from build123d import *

# Parameters (mm, degrees)
F1_DEPTH         = 19
F0_W             = 44.0000004768
F0_H             = 45.5000002384
F0_R             = 12
F2_DEPTH         = 2
F3_D             = 4
F5_DEPTH         = 50
F7_DEPTH         = 3
F8_D             = 4
F9_R             = 2
F10_R            = 34.4476203659
F10_W            = 47
F10_H            = 19
F6_W             = 47
F6_H             = 19
F11_DEPTH        = 3
F13_DEPTH        = 25
F14_D            = 4
F14_DEPTH        = 6
F14_TIP          = 1.2017212381
F14_ON_F12_D     = 4
F14_ON_F12_DEPTH = 6
F14_ON_F12_TIP   = 1.2017212381


# Not quite as in the source:
# - a feature names something its author has since deleted; it is built from what else it names


with BuildPart() as f1:
    # F0 (on Top) → F1 (new body)
    with BuildSketch(Plane.XY):
        Polygon((23.5, -23.5), (23.5, 23.5), (-23.5, 23.5), (-23.5, -23.5), (-22.0000002384, -23.5), (-22.0000002384, 22.0000002384), (22.0000002384, 22.0000002384), (22.0000002384, -23.5), align=None)
    extrude(amount=F1_DEPTH)

    # F0 (on Top) → F2 (join)
    with BuildSketch(Plane.XY):
        with Locations((0, -0.7499998808)):
            Rectangle(F0_W, F0_H)
        Circle(F0_R, mode=Mode.SUBTRACT)
    extrude(amount=F2_DEPTH)

    # F3 (through all)
    with Locations(Plane(origin=(0, 0, 0), x_dir=(1, 0, 0), z_dir=(0, 0, -1))):
        with Locations((-15.5, -15.5), (15.5, -15.5), (15.5, 15.5), (-15.5, 15.5)):
            Hole(F3_D / 2)

    # F4 (on face) → F5 (cut)
    with BuildSketch(Plane.YZ.offset(23.5)):
        Polygon((-23.5, 19), (-23.5, 2.1775800269), (17.5668895245, 19), align=None)
    extrude(amount=-F5_DEPTH, mode=Mode.SUBTRACT)

    # F6 (on face) → F7 (join)
    with BuildSketch(Plane(origin=(0, 23.5, 0), x_dir=(-1, 0, 0), z_dir=(0, 1, 0))):
        with BuildLine():
            Line((-23.5, 19), (-25.1444590574, 19))
            ThreePointArc((-25.1444590574, 19), (-28.6799929633, 17.5355339059), (-30.1444590574, 14))
            Line((-30.1444590574, 14), (-30.1444590574, 5))
            ThreePointArc((-30.1444590574, 5), (-28.6799929633, 1.4644660941), (-25.1444590574, 0))
            Line((-25.1444590574, 0), (-23.5, 0))
            Line((-23.5, 0), (-23.5, 19))
        make_face()
        with BuildLine():
            Line((24.0855421871, 19), (23.5, 19))
            Line((23.5, 19), (23.5, 0))
            Line((23.5, 0), (24.0855421871, 0))
            ThreePointArc((24.0855421871, 0), (27.621076093, 1.4644660941), (29.0855421871, 5))
            Line((29.0855421871, 5), (29.0855421871, 14))
            ThreePointArc((29.0855421871, 14), (27.621076093, 17.5355339059), (24.0855421871, 19))
        make_face()
    extrude(amount=-F7_DEPTH)

    # F8 (through all)
    with Locations(Plane(origin=(0, 23.5, 0), x_dir=(-1, 0, 0), z_dir=(0, 1, 0))):
        with Locations((-26.7366040498, 8.9737372473), (28.2633959502, 9.5)):
            Hole(F8_D / 2)

    # F9
    f9_edges = [f1.edges().sort_by_distance(p)[0] for p in [
        (22, 22, 10.5),
        (-22, 22, 10.5),
    ]]
    fillet(f9_edges, radius=F9_R)

    # F10 (on face) + F6 (on face) → F11 (join)
    with BuildSketch(Plane(origin=(0, 23.5, 0), x_dir=(-1, 0, 0), z_dir=(0, 1, 0))):
        with Locations((0, 19.7549201548)):
            Circle(F10_R)
        with Locations((0, 9.5)):
            Rectangle(F10_W, F10_H, mode=Mode.SUBTRACT)
    with BuildSketch(Plane(origin=(0, 23.5, 0), x_dir=(-1, 0, 0), z_dir=(0, 1, 0))):
        with Locations((0, 9.5)):
            Rectangle(F6_W, F6_H)
    extrude(amount=-F11_DEPTH)

    # F12 (on face) → F13 (cut)
    with BuildSketch(Plane(origin=(0, 23.5, 0), x_dir=(-1, 0, 0), z_dir=(0, 1, 0))):
        with BuildLine():
            ThreePointArc((-18.1099253817, 36.3759554919), (-20.9291093364, 32.8831264718), (-21.9364919731, 28.5090170817))
            Line((-21.9364919731, 28.5090170817), (-21.9364919731, 14.7631261498))
            Line((-21.9364919731, 14.7631261498), (21.9364919731, 14.7631261498))
            Line((21.9364919731, 14.7631261498), (21.9364919731, 28.5090170817))
            ThreePointArc((21.9364919731, 28.5090170817), (20.9291093364, 32.8831264718), (18.1099253817, 36.3759554919))
            Line((18.1099253817, 36.3759554919), (6.1734334086, 45.7428952702))
            ThreePointArc((6.1734334086, 45.7428952702), (0, 47.87595686), (-6.1734334086, 45.7428952702))
            Line((-6.1734334086, 45.7428952702), (-18.1099253817, 36.3759554919))
        make_face()
        with BuildLine():
            Line((28.2202352675, 0), (-28.2202352675, 0))
            ThreePointArc((-28.2202352675, 0), (0, -14.6927002111), (28.2202352675, 0))
        make_face()
    extrude(amount=-F13_DEPTH, mode=Mode.SUBTRACT)

    # F14
    with Locations(Plane(origin=(0, 23.5, 0), x_dir=(-1, 0, 0), z_dir=(0, 1, 0))):
        with Locations((-30.1444590574, 19), (-26.7366040498, 8.9737372473), (26.7366040498, 8.9737372473), (30.1444590574, 19)):
            Hole(F14_D / 2, depth=F14_DEPTH)
            with Locations((0, 0, -(F14_DEPTH + F14_TIP / 2))):  # 118° drill point
                Cone(0, F14_D / 2, F14_TIP, mode=Mode.SUBTRACT)

    # F14 on F12
    with Locations(Plane(origin=(0, 23.5, 0), x_dir=(-1, 0, 0), z_dir=(0, 1, 0))):
        with Locations((9.4067957252, 48.2378602028), (-9.4067957252, 48.2378602028)):
            Hole(F14_ON_F12_D / 2, depth=F14_ON_F12_DEPTH)
            with Locations((0, 0, -(F14_ON_F12_DEPTH + F14_ON_F12_TIP / 2))):  # 118° drill point
                Cone(0, F14_ON_F12_D / 2, F14_ON_F12_TIP, mode=Mode.SUBTRACT)


solid = f1.part
The model under review builds one solid part; all positions refer to its coordinate system, in mm. A direction names the side the tool comes from. Give positions to 0.01 mm unless a question says otherwise; leave off trailing zeros. Write each loop counter-clockwise with the first axis right and the second up, starting at its lowest first coordinate (ties: lowest second). Pieces come first, ordered by that corner, then holes. Notation, with made-up numbers: M 78,82.25 L 123,82.25 A23 ccw 123,99.25 Z; hole C -30,-3 d7. An arc over 180 degrees is marked long. One line per question, with ' | ' between items. Start each with the question number.
Item 1: We need section D-D on z = 24.5. Write out the cut boundary in (x, y).
Item 2: Wall thickness on line 1 (Y direction, x = -15.5, z = 0.45); line 2 (Y direction, x = -23.5, z = 39); line 3 (Z direction, x = -2, y = -18): over which ranges is each line inside the solid? List them lowest first. Write a range as from..to.
Item 3: For faces 3 (the flat face through (-5.2, -11, 2)), 4 (the cylindrical face through (-15.24, 13.517, 1.014)), 5 (the flat face through (0, -23.5, 1)), 6 (the flat face through (-23, 19, 19)), 7 (the cylindrical face through (-20.957, 22.021, 32.826)), list the 3-axis set-ups (+Z, -Z, +X, -X, +Y, -Y) from which the entire face can be reached by the end or side of a thin tool; tool diameter is ignored.
Item 4: For pin 1 (5 mm diameter, centred on x = -30.14, z = 19, fed in from -Y); pin 2 (15 mm diameter, centred on y = -8, z = 11, fed in from -X); pin 3 (21 mm diameter, centred on y = 1.5, z = 12.5, fed in from +X); pin 4 (2.5 mm diameter, centred on x = 15.5, y = -15.5, fed in from +Z), all flat-tipped, find the tip position at first contact; note any pin that passes through.
Item 5: We need section C-C on x = -19.5. Write out the cut boundary in (y, z), plus the area to 3 significant figures.
Item 6: Draft analysis for pull direction X (two halves, no side actions). For faces 1 (the flat face through (0, 23.5, 9)), 2 (the cylindrical face through (-11.99, 0.53, 0.99)), state which applies: released by +X, released by -X, zero draft, split by the parting line, or undercut.
Item 7: We need section B-B on y = -2. Write out the cut boundary in (x, z).
Item 8: We need section A-A on x = 0. Write out the cut boundary in (y, z).
Results found:
1) outline: M -34.12,20.5 L -21.94,20.5 L -21.94,23.5 L -34.12,23.5 Z; M 21.94,20.5 L 34.12,20.5 L 34.12,23.5 L 21.94,23.5 Z
2) line 1: y = -23.5..-17.5, -13.5..13.5, 17.5..23.5 | line 2: y = 20.5..23.5 | line 3: z = 0..2
3) face 3: +Z, -Y | face 4: +Z, -Z | face 5: +Z, -Z, +X, -X, -Y | face 6: +Z, +X, -X, -Y | face 7: +Y, -Y
4) pin 1: stops at y = 20.5 | pin 2: stops at x = -23.5 | pin 3: stops at x = 23.5 | pin 4: passes through
5) outline: M -23.5,0 L 23.5,0 L 23.5,14.76 L 20.5,14.76 L 20.5,2 L -23.5,2 Z; M 20.5,35.05 L 23.5,35.05 L 23.5,48.15 L 20.5,48.15 Z | area: 172 mm2
6) face 1: zero draft | face 2: undercut
7) outline: M -23.5,0 L -11.83,0 L -11.83,2 L -22,2 L -22,10.98 L -23.5,10.98 Z; M 11.83,0 L 23.5,0 L 23.5,10.98 L 22,10.98 L 22,2 L 11.83,2 Z
8) outline: M -23.5,0 L -12,0 L -12,2 L -23.5,2 Z; M 12,0 L 23.5,0 L 23.5,14.76 L 20.5,14.76 L 20.5,2 L 12,2 Z; M 20.5,47.88 L 23.5,47.88 L 23.5,54.2 L 20.5,54.2 Z
